Answer from the drawing. Dimensions are ordinates in mm from the lowest x, y and z of the part. Coordinates: 2 decimals unless noted, no trailing zeros. Write each loop counter-clockwise with the first axis right and the second up, starting at its lowest first coordinate (ties: lowest second). Pieces come first, ordered by that corner, then holes. Notation, with made-up numbers: (41, 62) -> (95, 62) arc R20 cw to (95, 89) -> close; hole circle Ø9 at (81, 83.25). An arc over 180 degrees is marked (long way). One line per item, written item: value. Start each with the question number.
1. Given P1, Ø1, axis at x = 31, y = 1, coming from the +Z side, flat-ended and moving along its own axis, determine where the tip first touches the part or whether it passes through.
2. Find section A-A, the plane y = 2. Write down the section's boundary in (x, z).
3. Find section B-B, the plane z = 22.5. State how many separate pieces and enclosed holes the cut face has, and give its area (3 significant figures).
4. Consider line 1 along X through (y, z) = (2.15, 22.5); line 2 along Z through (x, y) = (11.5, 2.65) (1 decimal); line 3 along X through (y, z) = (1.8, 5.5) (1 decimal). Determine where each line is inside the solid, lowest interval first.
5. For a pull along X with two mould halves and no side action, classify the marked faces 1, 2 and 3 as pulls with the +X half, pulls with the -X half, needs draft (parallel to the pull), parting line crosses it, or undercut.
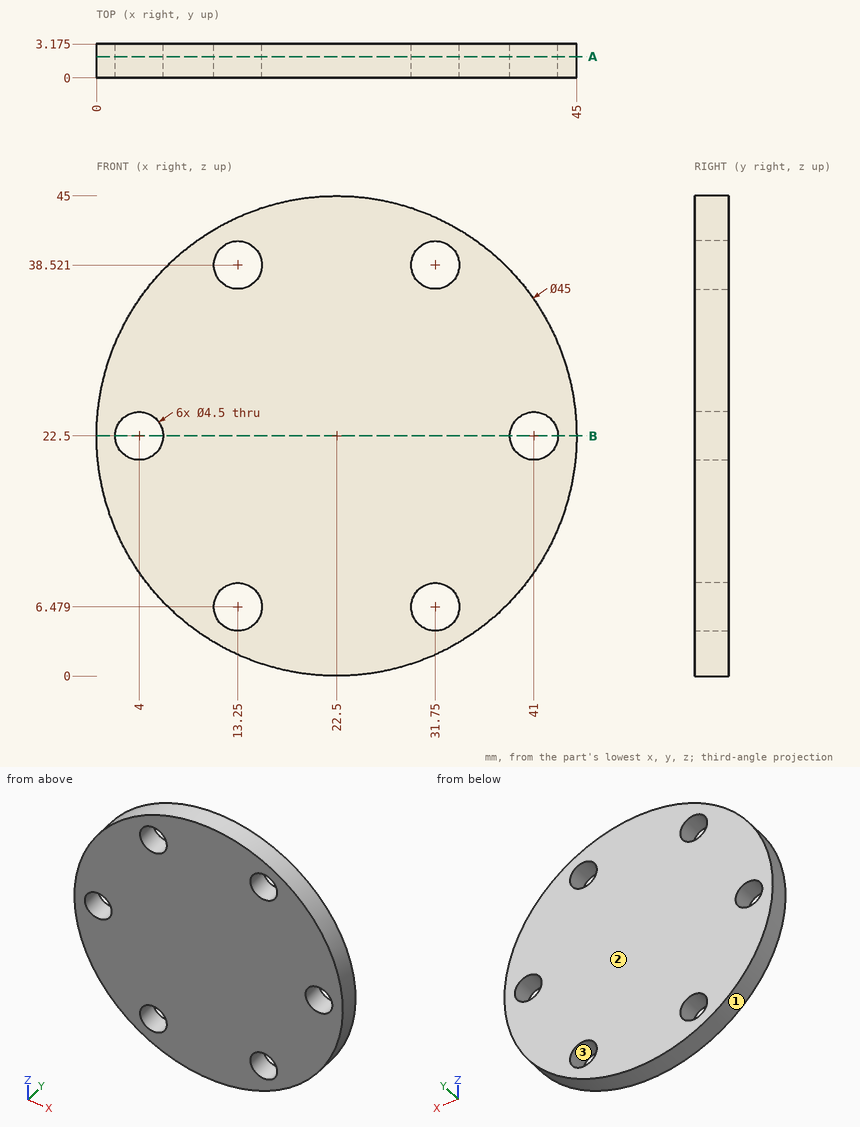
Answer block:
1. P1: stops at z = 43.53
2. outline: circle Ø45 at (22.5, 22.5); hole circle Ø4.5 at (4, 22.5); hole circle Ø4.5 at (13.25, 6.48); hole circle Ø4.5 at (13.25, 38.52); hole circle Ø4.5 at (31.75, 6.48); hole circle Ø4.5 at (31.75, 38.52); hole circle Ø4.5 at (41, 22.5)
3. separate pieces: 3
3. enclosed holes: 0
3. area: 114 mm2
4. line 1: x = 0 to 1.75, 6.25 to 38.75, 43.25 to 45
4. line 2: z = 2.9 to 5.1, 7.9 to 37.1, 39.9 to 42.1
4. line 3: x = 7.8 to 11.2, 15.3 to 29.7, 33.8 to 37.2
5. face 1: parting line crosses it
5. face 2: needs draft
5. face 3: undercut
